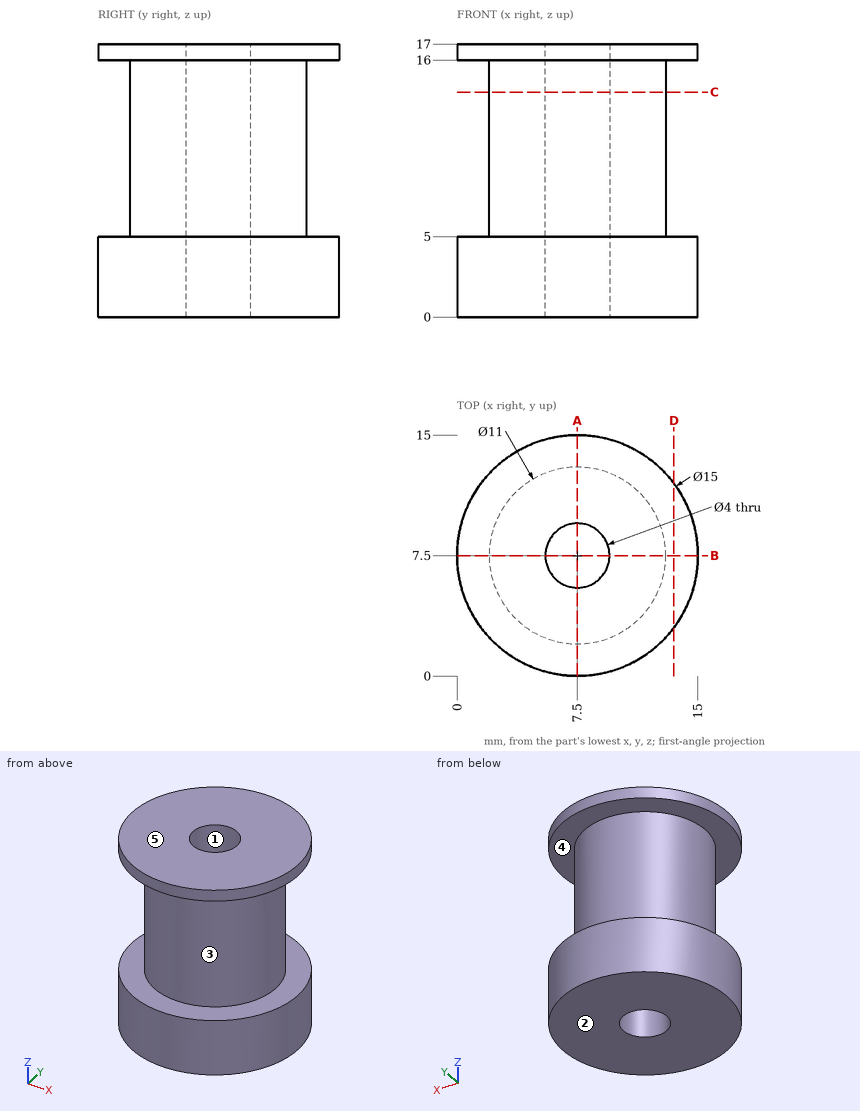
Study the drawing (mm; zero at the part's minimum x, y, z) and answer. A direction names the side the tool comes from. Give positions to 0.01 mm unless a question says otherwise; leave off trailing zeros. Order: outer loops, then holes, each group sorted by start corner. A loop starts at its lowest first (then second) coordinate and runs counter-clockwise, first axis right, second up. Notation, with made-up numbers: (-20, 14) - (13, 14) arc R25 ccw to (13, 51) - close; hole circle Ø8 at (5.25, 2). An arc over 180 degrees is marked (long way). Use one line per item in the form item = value. Start each with the question number.
(1) The mould has two halves that part along Z. Classify the marked faces 1, 2 and 3: released by +Z, released by -Z, zero draft, split by the parting line, or undercut.
(2) For the marked faces 4 and 5, determine the directions among +Z, -Z, +X, -X, +Y, -Y from which every point of the face is accessible in a straight line to the end or side of a thin tool.
(3) Consider line 1 (Y direction, x = 7.5, z = 6); line 2 (Z direction, x = 1.75, y = 12.25); line 3 (Y direction, x = 7, z = 11.75). Determine where each line is inside the solid, lowest interval first. Write a range as from..to.
(4) A cutting plane is placed at C-C, the plane z = 14. Write down the section's boundary in (x, y), then the cut area to 3 significant figures.
(5) A cutting plane is placed at D-D, the plane x = 13.5. Write down the section's boundary in (y, z).
(6) Flat-ended cylindrical pins translate along their axes: pin 1 Ø8 at (x, y) = (6.5, 9) entering from -Z; pin 2 Ø3 at (x, y) = (7.5, 7.5) entering from +Z; pin 3 Ø1 at (y, z) = (9.5, 7.5) entering from +X; pin 4 Ø8 at (y, z) = (8.5, 9.5) entering from -X. Find the tip coordinate at first contact, or state that the pin passes through.
(7) A cutting plane is placed at A-A, the plane x = 7.5. Write down the section's boundary in (y, z), then the cut area to 3 significant figures.
Ans:
q1.face_1 = zero draft
q1.face_2 = released by -Z
q1.face_3 = undercut
q2.face_4 = none
q2.face_5 = +Z, +X, -X, +Y, -Y
q3.line_1 = 2..5.5, 9.5..13
q3.line_2 = 0..5, 16..17
q3.line_3 = 2.02..5.56, 9.44..12.98
q4.outline = circle Ø11 at (7.5, 7.5); hole circle Ø4 at (7.5, 7.5)
q4.area = 82.5 mm^2
q5.outline = (3, 0) - (12, 0) - (12, 5) - (3, 5) - close; (3, 16) - (12, 16) - (12, 17) - (3, 17) - close
q6.pin_1 = 0
q6.pin_2 = through
q6.pin_3 = 12.79
q6.pin_4 = 2
q7.outline = (0, 0) - (5.5, 0) - (5.5, 17) - (0, 17) - (0, 16) - (2, 16) - (2, 5) - (0, 5) - close; (9.5, 0) - (15, 0) - (15, 5) - (13, 5) - (13, 16) - (15, 16) - (15, 17) - (9.5, 17) - close
q7.area = 143 mm^2
